```python
from build123d import *

# Parameters (mm, degrees)
SKETCH1_W           = 50.8
SKETCH1_H           = 25.4
SKETCH1_W_2         = 44.45
SKETCH1_H_2         = 19.05
BOSS_EXTRUDE1_DEPTH = 222.25
SKETCH3_R           = 2.15265
SKETCH3_R_2         = 2.159
CUT_EXTRUDE2_DEPTH  = 51.8
SKETCH4_R           = 2.4892
CUT_EXTRUDE3_DEPTH  = 51.8
SKETCH5_R           = 2.4892
CUT_EXTRUDE4_DEPTH  = 26.4


with BuildPart() as part:
    # Sketch1 → Boss-Extrude1 (new body, symmetric)
    with BuildSketch(Plane.XY):
        Rectangle(SKETCH1_W, SKETCH1_H)
        Rectangle(SKETCH1_W_2, SKETCH1_H_2, mode=Mode.SUBTRACT)
    extrude(amount=BOSS_EXTRUDE1_DEPTH, both=True)

    # Sketch3 → Cut-Extrude2 (cut, through all)
    with BuildSketch(Plane(origin=(25.4, 0, 0), x_dir=(0, 0, -1), z_dir=(1, 0, 0))):
        with Locations((-215.9, 0)):
            Circle(SKETCH3_R)
        with Locations((-190.5, 0)):
            Circle(SKETCH3_R)
        with Locations((-165.1, 0)):
            Circle(SKETCH3_R)
        with Locations((215.9, 0)):
            Circle(SKETCH3_R_2)
        with Locations((190.5, 0)):
            Circle(SKETCH3_R_2)
        with Locations((165.1, 0)):
            Circle(SKETCH3_R_2)
    extrude(amount=-CUT_EXTRUDE2_DEPTH, mode=Mode.SUBTRACT)

    # Sketch4 → Cut-Extrude3 (cut, through all)
    with BuildSketch(Plane(origin=(25.4, 0, 0), x_dir=(0, 0, -1), z_dir=(1, 0, 0))):
        with Locations((-139.7, 0)):
            Circle(SKETCH4_R)
        with Locations((-127, 0)):
            Circle(SKETCH4_R)
        with Locations((-114.3, 0)):
            Circle(SKETCH4_R)
        with Locations((-101.6, 0)):
            Circle(SKETCH4_R)
        with Locations((-88.9, 0)):
            Circle(SKETCH4_R)
        with Locations((-76.2, 0)):
            Circle(SKETCH4_R)
        with Locations((-63.5, 0)):
            Circle(SKETCH4_R)
        with Locations((-50.8, 0)):
            Circle(SKETCH4_R)
        with Locations((-38.1, 0)):
            Circle(SKETCH4_R)
        with Locations((-25.4, 0)):
            Circle(SKETCH4_R)
        with Locations((-12.7, 0)):
            Circle(SKETCH4_R)
        Circle(SKETCH4_R)
        with Locations((12.7, 0)):
            Circle(SKETCH4_R)
        with Locations((25.4, 0)):
            Circle(SKETCH4_R)
        with Locations((38.1, 0)):
            Circle(SKETCH4_R)
        with Locations((50.8, 0)):
            Circle(SKETCH4_R)
        with Locations((63.5, 0)):
            Circle(SKETCH4_R)
        with Locations((76.2, 0)):
            Circle(SKETCH4_R)
        with Locations((88.9, 0)):
            Circle(SKETCH4_R)
        with Locations((101.6, 0)):
            Circle(SKETCH4_R)
        with Locations((114.3, 0)):
            Circle(SKETCH4_R)
        with Locations((127, 0)):
            Circle(SKETCH4_R)
        with Locations((139.7, 0)):
            Circle(SKETCH4_R)
    extrude(amount=-CUT_EXTRUDE3_DEPTH, mode=Mode.SUBTRACT)

    # Sketch5 → Cut-Extrude4 (cut, through all)
    with BuildSketch(Plane.XZ.offset(12.7)):
        with Locations((-12.7, 133.35)):
            Circle(SKETCH5_R)
        with Locations((0, 133.35)):
            Circle(SKETCH5_R)
        with Locations((12.7, 133.35)):
            Circle(SKETCH5_R)
        with Locations((12.7, -133.35)):
            Circle(SKETCH5_R)
        with Locations((0, -133.35)):
            Circle(SKETCH5_R)
        with Locations((-12.7, -133.35)):
            Circle(SKETCH5_R)
        with Locations((-12.7, 44.45)):
            Circle(SKETCH5_R)
        with Locations((0, 44.45)):
            Circle(SKETCH5_R)
        with Locations((12.7, 44.45)):
            Circle(SKETCH5_R)
        with Locations((12.7, 31.75)):
            Circle(SKETCH5_R)
        with Locations((0, 31.75)):
            Circle(SKETCH5_R)
        with Locations((-12.7, 31.75)):
            Circle(SKETCH5_R)
        with Locations((12.7, 19.05)):
            Circle(SKETCH5_R)
        with Locations((0, 19.05)):
            Circle(SKETCH5_R)
        with Locations((-12.7, 19.05)):
            Circle(SKETCH5_R)
        with Locations((12.7, 6.35)):
            Circle(SKETCH5_R)
        with Locations((0, 6.35)):
            Circle(SKETCH5_R)
        with Locations((-12.7, 6.35)):
            Circle(SKETCH5_R)
        with Locations((12.7, -6.35)):
            Circle(SKETCH5_R)
        with Locations((0, -6.35)):
            Circle(SKETCH5_R)
        with Locations((-12.7, -6.35)):
            Circle(SKETCH5_R)
        with Locations((12.7, -19.05)):
            Circle(SKETCH5_R)
        with Locations((0, -19.05)):
            Circle(SKETCH5_R)
        with Locations((-12.7, -19.05)):
            Circle(SKETCH5_R)
        with Locations((12.7, -31.75)):
            Circle(SKETCH5_R)
        with Locations((0, -31.75)):
            Circle(SKETCH5_R)
        with Locations((-12.7, -31.75)):
            Circle(SKETCH5_R)
        with Locations((12.7, -44.45)):
            Circle(SKETCH5_R)
        with Locations((0, -44.45)):
            Circle(SKETCH5_R)
        with Locations((-12.7, -44.45)):
            Circle(SKETCH5_R)
    extrude(amount=-CUT_EXTRUDE4_DEPTH, mode=Mode.SUBTRACT)


solid = part.part
```
Work out the finished part from the listing and answer in its coordinate system (mm). A direction names the side the tool comes from. Give positions to 0.01 mm unless a question says otherwise; leave off trailing zeros. Order: outer loops, then holes, each group sorted by start corner. A loop starts at its lowest first (then second) coordinate and runs counter-clockwise, first axis right, second up. Notation, with made-up numbers: (24, 5) -> (44, 5) arc R25 ccw to (44, 21) -> close; hole circle Ø1 at (74, 7). An arc over 180 degrees is marked (long way). Answer as CSV lines item,"result". Start each with the question number.
(1) Which of the six approach directions +Z, -Z, +X, -X, +Y, -Y give full straight-line access (tool end or side, diameter ignored) to faces 1 (the flat face through (0, 10, -222.25)), 2 (the flat face through (0, 9.525, 3))?
(2) For a pull along Y with two mould halves and no side action, classify faces 3 (the flat face through (22.225, 0, 3)), 4 (the flat face through (0, 12.7, 3)), 5 (the flat face through (0, -12.7, 3)), 6 (the flat face through (0, 10, 222.25)) as released by +Y, released by -Y, zero draft, split by the parting line, or undercut.
(3) Section B-B, the plane x = -6.5 is taken. Write down the section's boundary in (y, z) (3 decimals).
(4) Section A-A, the plane z = -171.5 is taken. Write down the section's boundary in (x, y) (3 decimals).
(5) Consider line 1 along Y through (x, z) = (3.5, -152) (3 decimals); line 2 along X through (y, z) = (-8.75, -3) (3 decimals); line 3 along Y through (x, z) = (24.7, 76.2). Determine where each line is inside the solid, lowest interval first.
Entries:
1,face 1,"-Z, +X, -X, +Y, -Y"
1,face 2,"+Z, -Z"
2,face 3,"undercut"
2,face 4,"released by +Y"
2,face 5,"released by -Y"
2,face 6,"zero draft"
3,outline,"(-12.7, -222.25) -> (-9.525, -222.25) -> (-9.525, 222.25) -> (-12.7, 222.25) -> close; (9.525, -222.25) -> (12.7, -222.25) -> (12.7, 222.25) -> (9.525, 222.25) -> close"
4,outline,"(-25.4, -12.7) -> (25.4, -12.7) -> (25.4, 12.7) -> (-25.4, 12.7) -> close; hole (-22.225, -9.525) -> (22.225, -9.525) -> (22.225, 9.525) -> (-22.225, 9.525) -> close"
5,line 1,"-12.7 to -9.525, 9.525 to 12.7"
5,line 2,"-25.4 to -22.225, 22.225 to 25.4"
5,line 3,"-12.7 to -2.49, 2.49 to 12.7"
